```python
from build123d import *

# Parameters (mm, degrees)
F0_R     = 0.875
F1_DEPTH = 2
F4_DEPTH = 2.5
F6_DEPTH = 25.4913661255
F7_R     = 5
F8_R     = 3
F9_SIZE  = 1.25


with BuildPart() as f1:
    # F0 (on Top) → F1 (new body)
    with BuildSketch(Plane.XY):
        Polygon((14.75, 0), (0, 0), (-14.75, 0), (-14.75, -5.25), (-10.75, -5.25), (-10.75, -16.5), (0, -16.5), (10.75, -16.5), (10.75, -5.25), (14.75, -5.25), align=None)
        with Locations((-7, -7)):
            Circle(F0_R, mode=Mode.SUBTRACT)
        with Locations((0, -7)):
            Circle(F0_R, mode=Mode.SUBTRACT)
        with Locations((7, -7)):
            Circle(F0_R, mode=Mode.SUBTRACT)
    extrude(amount=F1_DEPTH)

    # F3 (on face) → F4 (join)
    with BuildSketch(Plane(origin=(0, 0, 0), x_dir=(-1, 0, 0), z_dir=(0, 0.7660444431, -0.6427876097))):
        with BuildLine():
            Line((-14.75, 0), (14.75, 0))
            Line((14.75, 0), (14.75, 1.3812757004))
            ThreePointArc((14.75, 1.3812757004), (15.2754453264, 2.7324561156), (16.5756885145, 3.3736650966))
            Line((16.5756885145, 3.3736650966), (24.147387942, 4.0361029601))
            ThreePointArc((24.147387942, 4.0361029601), (24.9815296917, 4.1810344722), (25.7792604037, 4.464624516))
            Line((25.7792604037, 4.464624516), (39.0676511754, 10.5))
            ThreePointArc((39.0676511754, 10.5), (41.2034661814, 12.3448936136), (42, 15.0524519346))
            Line((42, 15.0524519346), (42, 16.5491437132))
            ThreePointArc((42, 16.5491437132), (40.7746857814, 19.8281294179), (37.6993010994, 21.5))
            Line((37.6993010994, 21.5), (20, 24))
            Line((20, 24), (0, 24))
            Line((0, 24), (-20, 24))
            Line((-20, 24), (-37.6993010994, 21.5))
            ThreePointArc((-37.6993010994, 21.5), (-40.7746857814, 19.8281294179), (-42, 16.5491437132))
            Line((-42, 16.5491437132), (-42, 15.0524519346))
            ThreePointArc((-42, 15.0524519346), (-41.2034661814, 12.3448936136), (-39.0676511754, 10.5))
            Line((-39.0676511754, 10.5), (-25.7792604037, 4.464624516))
            ThreePointArc((-25.7792604037, 4.464624516), (-24.9815296917, 4.1810344722), (-24.147387942, 4.0361029601))
            Line((-24.147387942, 4.0361029601), (-16.5756885145, 3.3736650966))
            ThreePointArc((-16.5756885145, 3.3736650966), (-15.2754453264, 2.7324561156), (-14.75, 1.3812757004))
            Line((-14.75, 1.3812757004), (-14.75, 0))
        make_face()
    extrude(amount=-F4_DEPTH)

    # F5 (on face) → F6 (cut, through all)
    with BuildSketch(Plane(origin=(0, 0, 0), x_dir=(-1, 0, 0), z_dir=(0, 0.7660444431, -0.6427876097))):
        with BuildLine():
            Line((-21.098955464, 20.8149952552), (-37.2797204398, 18.5294862279))
            ThreePointArc((-37.2797204398, 18.5294862279), (-38.5098743126, 17.8607379951), (-39, 16.5491437132))
            Line((-39, 16.5491437132), (-39, 15.0524519346))
            ThreePointArc((-39, 15.0524519346), (-38.6813864726, 13.9694286062), (-37.8270604702, 13.2314711608))
            Line((-37.8270604702, 13.2314711608), (-26.8148956657, 8.2299212644))
            Line((-26.8148956657, 8.2299212644), (-21.098955464, 20.8149952552))
        make_face()
        with BuildLine():
            Line((-12.2691561683, 21), (-18.2691561683, 21))
            Line((-18.2691561683, 21), (-24.5386696984, 7.1960956767))
            ThreePointArc((-24.5386696984, 7.1960956767), (-24.2195774136, 7.0826596592), (-23.8859207138, 7.0246870544))
            Line((-23.8859207138, 7.0246870544), (-15.0312071638, 6.25))
            Line((-15.0312071638, 6.25), (-6.732866085, 6.25))
            Line((-6.732866085, 6.25), (-12.2691561683, 21))
        make_face()
        with BuildLine():
            Line((18.2691561683, 21), (12.2691561683, 21))
            Line((12.2691561683, 21), (6.732866085, 6.25))
            Line((6.732866085, 6.25), (15.0312071638, 6.25))
            Line((15.0312071638, 6.25), (23.8859207138, 7.0246870544))
            ThreePointArc((23.8859207138, 7.0246870544), (24.2195774136, 7.0826596592), (24.5386696984, 7.1960956767))
            Line((24.5386696984, 7.1960956767), (18.2691561683, 21))
        make_face()
        with BuildLine():
            Line((37.2797204398, 18.5294862279), (21.098955464, 20.8149952552))
            Line((21.098955464, 20.8149952552), (26.8148956657, 8.2299212644))
            Line((26.8148956657, 8.2299212644), (37.8270604702, 13.2314711608))
            ThreePointArc((37.8270604702, 13.2314711608), (38.6813864726, 13.9694286062), (39, 15.0524519346))
            Line((39, 15.0524519346), (39, 16.5491437132))
            ThreePointArc((39, 16.5491437132), (38.5098743126, 17.8607379951), (37.2797204398, 18.5294862279))
        make_face()
    extrude(amount=-F6_DEPTH, mode=Mode.SUBTRACT)

    # F7 (call 1 of 2: OpenCascade refuses the feature's edges together)
    f7_edges = [f1.edges().sort_by_distance(p)[0] for p in [
        (0, -1.585319, 2),
    ]]
    fillet(f7_edges, radius=F7_R)

    # F7#2 (call 2 of 2)
    f7_2_edges = [f1.edges().sort_by_distance(p)[0] for p in [
        (0, 0, 0),
    ]]
    fillet(f7_2_edges, radius=F7_R)

    # F8
    f8_edges = [f1.edges().sort_by_distance(p)[0] for p in [
        (-21.098955, 12.422065, 16.748696),
        (-26.814896, 4.332536, 7.10797),
        (-24.53867, 3.668006, 6.316014),
        (-6.732866, 3.059867, 5.591262),
        (-12.269156, 12.540984, 16.890418),
        (-18.269156, 12.540984, 16.890418),
        (12.269156, 12.540984, 16.890418),
        (18.269156, 12.540984, 16.890418),
        (24.53867, 3.668006, 6.316014),
        (6.732866, 3.059867, 5.591262),
        (26.814896, 4.332536, 7.10797),
        (21.098955, 12.422065, 16.748696),
    ]]
    fillet(f8_edges, radius=F8_R)

    # F9
    f9_edges = [f1.edges().sort_by_distance(p)[0] for p in [
        (-7.875, -7, 0),
        (-0.875, -7, 0),
        (6.125, -7, 0),
    ]]
    chamfer(f9_edges, length=F9_SIZE)


solid = f1.part
```
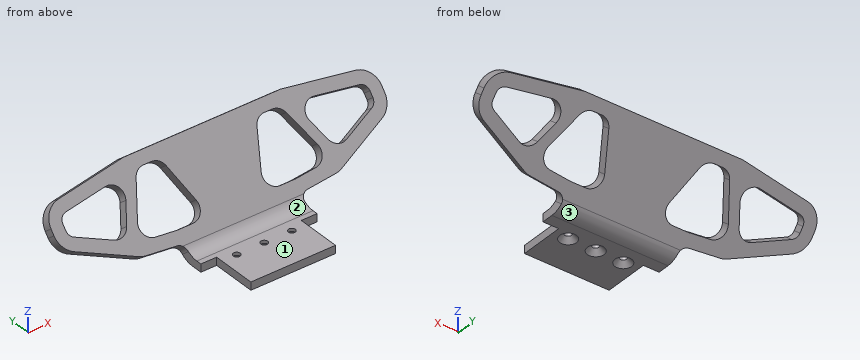
Geometry check sheet. Reference: the model listing, model coordinates, mm. Face numbers are marked on the shaded views. Give positions to 0.01 mm unless a question says otherwise; leave off trailing zeros. Write each loop counter-clockwise with the first axis right and the second up, starting at its lowest first coordinate (ties: lowest second). Pieces come first, ordered by that corner, then holes.
1) Material ranges on L1, parallel to X at y = 8.5, z = 13.75; L2, parallel to Y at x = 0, z = 1.4 (3 decimals); L3, parallel to Z at x = 8.5, y = -8.5, recorded low to high.
2) Release check for a two-part mould opening along Y. For the marked faces 1, 2 and 3 record: pulls with the +Y half, pulls with the -Y half, needs draft (parallel to the pull), parting line crosses it, or undercut.
3) Section check D-D, the plane x = 32. Record the boundary of the cut face in (y, z).
4) Section check C-C, the plane x = 4. Record the boundary of the cut face in (y, z), and give its area (3 significant figures).
5) Gauge pin test, flat ends, axial feed: pin 1 (1 mm diameter, centred on x = -12, z = 1, fed in from -Y); pin 2 (2 mm diameter, centred on x = -7, y = -7, fed in from +Z); pin 3 (3 mm diameter, centred on y = -12, z = 3, fed in from -X). Record the tip position at first contact, or that the pin passes through.
6) Section check B-B, the plane y = -7. Record the boundary of the cut face in (x, z) (3 decimals), and give its area (3 significant figures).
7) Section check A-A, the plane x = -7. Record the boundary of the cut face in (y, z) (3 decimals).
Computed:
1. L1: x = -42 to -39, -23.29 to -20.54, -10.39 to 10.39, 20.54 to 23.29, 39 to 42
1. L2: y = -16.5 to -7.875, -6.125 to 1.138
1. L3: z = 0 to 2
2. face 1: needs draft
2. face 2: pulls with the -Y half
2. face 3: pulls with the +Y half
3. outline: (2.77, 7.19) - (4.69, 5.58) - (6.8, 8.11) - (4.89, 9.72) - close; (10.47, 16.37) - (12.39, 14.77) - (14.34, 17.09) - (12.42, 18.69) - close
4. outline: (-16.5, 0) - (-2.33, 0) arc R5 ccw to (1.5, 1.79) - (15.43, 18.39) - (13.51, 19.99) - (-0.09, 3.79) arc R5 cw to (-3.92, 2) - (-16.5, 2) - close
4. area: 90.8 mm2
5. pin 1: stops at y = -5.25
5. pin 2: stops at z = 2
5. pin 3: stops at x = -10.75
6. outline: (-10.75, 0) - (-9.125, 0) - (-7.875, 1.25) - (-7.875, 2) - (-10.75, 2) - close; (-6.125, 1.25) - (-4.875, 0) - (-2.125, 0) - (-0.875, 1.25) - (-0.875, 2) - (-6.125, 2) - close; (0.875, 1.25) - (2.125, 0) - (4.875, 0) - (6.125, 1.25) - (6.125, 2) - (0.875, 2) - close; (7.875, 1.25) - (9.125, 0) - (10.75, 0) - (10.75, 2) - (7.875, 2) - close
6. area: 27.8 mm2
7. outline: (-16.5, 0) - (-9.125, 0) - (-7.875, 1.25) - (-7.875, 2) - (-16.5, 2) - close; (-6.125, 1.25) - (-4.875, 0) - (-2.332, 0) arc R5 ccw to (1.499, 1.786) - (15.427, 18.385) - (13.512, 19.992) - (-0.087, 3.786) arc R5 cw to (-3.917, 2) - (-6.125, 2) - close
